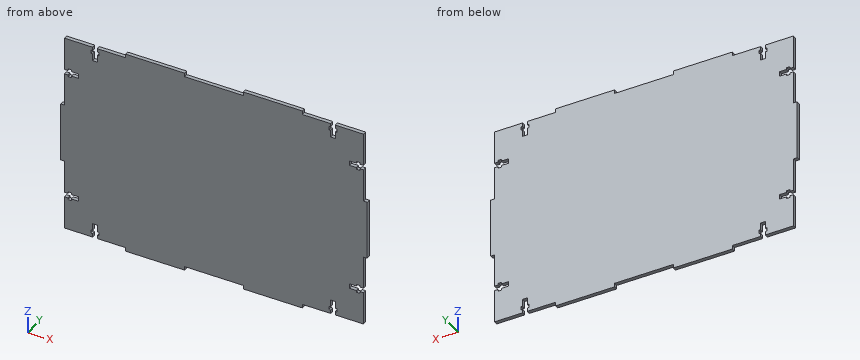
```python
from build123d import *

# Parameters (mm, degrees)
BOSS_EXTRUDE1_DEPTH     = 1.5875
CUT_EXTRUDE1_DEPTH      = 1
CUT_EXTRUDE1_DEPTH_BACK = 4.175


with BuildPart() as part:
    # Sketch1 → Boss-Extrude1 (new body, symmetric)
    with BuildSketch(Plane(origin=(0, 0, 0), x_dir=(1, 0, 0), z_dir=(0, 1, 0))):
        Polygon((55, 3.175), (55, 0), (105, 0), (105, 3.175), (155, 3.175), (155, 0), (205, 0), (205, 3.175), (256.825, 3.175), (256.825, 63), (260, 63), (260, 113), (256.825, 113), (256.825, 172.825), (205, 172.825), (205, 176), (155, 176), (155, 172.825), (105, 172.825), (105, 176), (55, 176), (55, 172.825), (3.175, 172.825), (3.175, 113), (0, 113), (0, 63), (3.175, 63), (3.175, 3.175), align=None)
    extrude(amount=BOSS_EXTRUDE1_DEPTH, both=True)

    # Sketch3 → Cut-Extrude1 (cut, two sides)
    with BuildSketch(Plane(origin=(0, 1.5875, 0), x_dir=(1, 0, 0), z_dir=(0, 1, 0))) as cut_extrude1_sk:
        Polygon((228.9125, 3.175), (232.9125, 3.175), (232.9125, 6.175), (234.4125, 6.175), (234.4125, 9.175), (232.9125, 9.175), (232.9125, 15.175), (228.9125, 15.175), (228.9125, 9.175), (227.4125, 9.175), (227.4125, 6.175), (228.9125, 6.175), align=None)
        Polygon((253.825, 31.0875), (256.825, 31.0875), (256.825, 35.0875), (253.825, 35.0875), (253.825, 36.5875), (250.825, 36.5875), (250.825, 35.0875), (244.825, 35.0875), (244.825, 31.0875), (250.825, 31.0875), (250.825, 29.5875), (253.825, 29.5875), align=None)
        Polygon((253.825, 140.9125), (256.825, 140.9125), (256.825, 144.9125), (253.825, 144.9125), (253.825, 146.4125), (250.825, 146.4125), (250.825, 144.9125), (244.825, 144.9125), (244.825, 140.9125), (250.825, 140.9125), (250.825, 139.4125), (253.825, 139.4125), align=None)
        Polygon((232.9125, 169.825), (232.9125, 172.825), (228.9125, 172.825), (228.9125, 169.825), (227.4125, 169.825), (227.4125, 166.825), (228.9125, 166.825), (228.9125, 160.825), (232.9125, 160.825), (232.9125, 166.825), (234.4125, 166.825), (234.4125, 169.825), align=None)
        Polygon((25.5875, 169.825), (25.5875, 166.825), (27.0875, 166.825), (27.0875, 160.825), (31.0875, 160.825), (31.0875, 166.825), (32.5875, 166.825), (32.5875, 169.825), (31.0875, 169.825), (31.0875, 172.825), (27.0875, 172.825), (27.0875, 169.825), align=None)
        Polygon((6.175, 144.9125), (3.175, 144.9125), (3.175, 140.9125), (6.175, 140.9125), (6.175, 139.4125), (9.175, 139.4125), (9.175, 140.9125), (15.175, 140.9125), (15.175, 144.9125), (9.175, 144.9125), (9.175, 146.4125), (6.175, 146.4125), align=None)
        Polygon((6.175, 35.0875), (3.175, 35.0875), (3.175, 31.0875), (6.175, 31.0875), (6.175, 29.5875), (9.175, 29.5875), (9.175, 31.0875), (15.175, 31.0875), (15.175, 35.0875), (9.175, 35.0875), (9.175, 36.5875), (6.175, 36.5875), align=None)
        Polygon((27.0875, 6.175), (27.0875, 3.175), (31.0875, 3.175), (31.0875, 6.175), (32.5875, 6.175), (32.5875, 9.175), (31.0875, 9.175), (31.0875, 15.175), (27.0875, 15.175), (27.0875, 9.175), (25.5875, 9.175), (25.5875, 6.175), align=None)
    extrude(amount=CUT_EXTRUDE1_DEPTH, mode=Mode.SUBTRACT)
    extrude(cut_extrude1_sk.sketch, amount=-CUT_EXTRUDE1_DEPTH_BACK, mode=Mode.SUBTRACT)


solid = part.part
```
Geometry: final body of the model. Coordinates: model frame, mm. Round coordinates to 2 decimals unless told otherwise and drop trailing zeros. Loops run counter-clockwise (first coordinate to the right, second up) from the corner with the lowest first, then second, coordinate; pieces in that order, holes last. Notation, with made-up numbers: (-28, -4.5) -> (-7, -4.5) arc R8 cw to (-7, 2.5) -> close; hole circle Ø11 at (-23, 38). An arc over 180 degrees is marked (long way). Write each question's results on one line, items separated by ' | '.
Item 1: Cut plane A-A on z = -21. Return the cut outline in (x, y) (1 decimal), and give its area (3 significant figures).
Answers below:
outline: (3.2, -1.6) -> (256.8, -1.6) -> (256.8, 1.6) -> (3.2, 1.6) -> close | area: 805 mm²
Item 2: Line query: probe 1 along X at (y, z) = (0.05, -12.5) (1 decimal); probe 2 along Z at (x, y) = (245, -0.6) (1 decimal); probe 3 along Z at (x, y) = (228, -0.55) (3 decimals). Output: solid intervals per line, ascending. Write a range as [from, to].
Answers below:
probe 1: x = [3.2, 27.1], [31.1, 228.9], [232.9, 256.8] | probe 2: z = [-172.8, -144.9], [-140.9, -35.1], [-31.1, -3.2] | probe 3: z = [-172.825, -169.825], [-166.825, -9.175], [-6.175, -3.175]
Item 3: Cut plane B-B on x = 48.5. Return the cut outline in (y, z) (1 decimal), and give its area (3 significant figures).
Answers below:
outline: (-1.6, -172.8) -> (1.6, -172.8) -> (1.6, -3.2) -> (-1.6, -3.2) -> close | area: 539 mm²
Item 4: Pin query (flat end, axial travel): pin 1 Ø1.6 at (y, z) = (-0.5, -122) entering from -X (3 decimals); pin 2 Ø1.6 at (x, y) = (231, 0.5) entering from -Z (3 decimals); pin 3 Ø1.6 at (y, z) = (0, -123.5) entering from +X (3 decimals). Return the tip coordinate at first contact, or that it passes through.
Answers below:
pin 1: stops at x = 3.175 | pin 2: stops at z = -160.825 | pin 3: stops at x = 256.825
